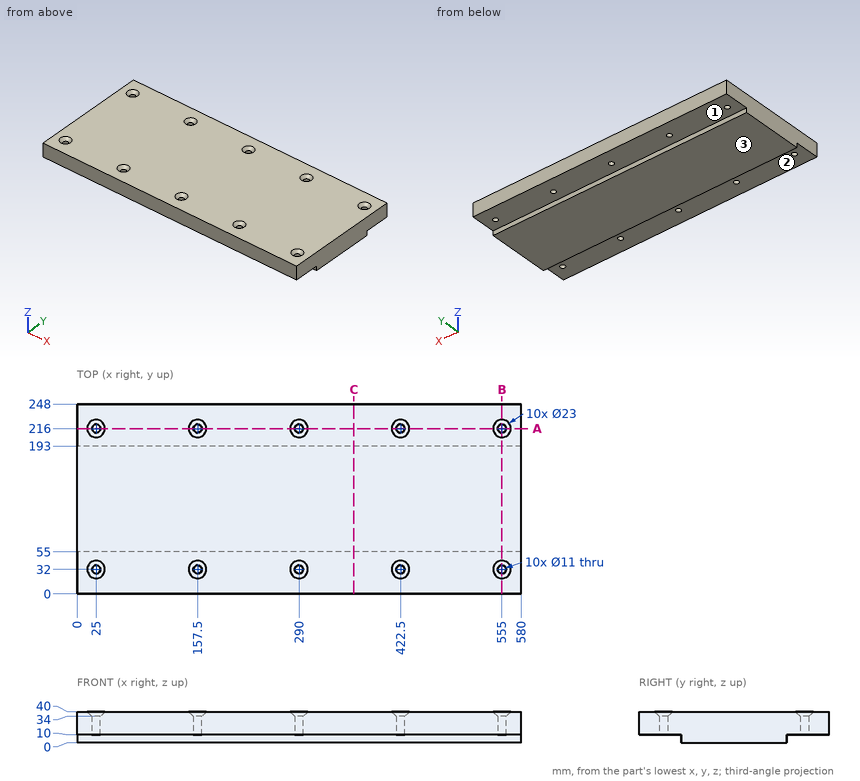
Answer from the drawing. Dimensions are ordinates in mm from the lowest x, y and z of the part. A direction names the side the tool comes from. Coordinates: 2 decimals unless noted, no trailing zeros. Write each loop counter-clockwise with the first axis right and the second up, starting at its lowest first coordinate (ties: lowest second). Pieces come first, ordered by that corner, then holes. Notation, with made-up numbers: M -31.5,28.25 L 26.5,28.25 A28 ccw 26.5,46.25 Z; hole C 82.25,78.25 d1. An arc over 180 degrees is marked long. Write item = value, one per line.
1. For the marked faces 1, 2 and 3, determine the directions among +Z, -Z, +X, -X, +Y, -Y from which every point of the face is accessible in a straight line to the end or side of a thin tool.
Solution:
face_1 = -Z, +X, -X, +Y
face_2 = -Z, +X, -X, -Y
face_3 = -Z, +X, -X, +Y, -Y
2. The part is cut by section C-C (x = 361.5). Determine the outline of the cut face in (y, z).
Solution:
outline = M 0,10 L 55,10 L 55,0 L 193,0 L 193,10 L 248,10 L 248,40 L 0,40 Z
3. Straight lines are drawn through the part: line 1 (X direction, y = 32, z = 22.75); line 2 (Y direction, x = 555, z = 26.5); line 3 (X direction, y = 30.5, z = 28). For each, find the intervals that lie inside material, in ascending order. Write a range as from..to.
Solution:
line_1 = 0..19.5, 30.5..152, 163..284.5, 295.5..417, 428..549.5, 560.5..580
line_2 = 0..26.5, 37.5..210.5, 221.5..248
line_3 = 0..19.71, 30.29..152.21, 162.79..284.71, 295.29..417.21, 427.79..549.71, 560.29..580
4. Flat-ended cylindrical pins translate along their axes: pin 1 (12.5 mm diameter, centred on x = 422.5, y = 216, fed in from +Z); pin 2 (11 mm diameter, centred on x = 329.5, z = 3.5, fed in from +Y); pin 3 (14.5 mm diameter, centred on x = 422.5, y = 32, fed in from +Z). Find the tip coordinate at first contact, or state that the pin passes through.
Solution:
pin_1 = 34.75
pin_2 = 193
pin_3 = 35.75
5. The part is cut by section B-B (x = 555). Determine the outline of the cut face in (y, z).
Solution:
outline = M 0,10 L 26.5,10 L 26.5,34 L 20.5,40 L 0,40 Z; M 37.5,10 L 55,10 L 55,0 L 193,0 L 193,10 L 210.5,10 L 210.5,34 L 204.5,40 L 43.5,40 L 37.5,34 Z; M 221.5,10 L 248,10 L 248,40 L 227.5,40 L 221.5,34 Z
6. The part is cut by section A-A (y = 216). State how many separate pieces and enclosed holes the cut face has, then the cut area to 3 significant figures.
Solution:
separate_pieces = 6
enclosed_holes = 0
area = 15,600 mm2
